Can you work these out from the model? Positions are in its coordinate system, mm. Face numbers are marked on the shaded views. A direction names the side the tool comes from. Round coordinates to 2 decimals unless told otherwise and drop trailing zeros. Loops run counter-clockwise (first coordinate to the right, second up) from the corner with the lowest first, then second, coordinate; pieces in that order, holes last. Notation, with made-up numbers: (75, -19.75) -> (96, -19.75) arc R20 ccw to (96, 13.25) -> close; hole circle Ø4 at (19.5, 16.25). An arc over 180 degrees is marked (long way). Write item = value, one per line.
from build123d import *

# Parameters (mm, degrees)
SKETCH2_R          = 3
EXTRUDE1_DEPTH     = 10
SKETCH3_R          = 5
EXTRUDE2_DEPTH     = 6
CUT_EXTRUDE1_DEPTH = 6
FILLET1_R          = 0.5
CHAMFER1_SIZE      = 0.5


with BuildPart() as part:
    # Sketch2 → Extrude1 (new body)
    with BuildSketch(Plane.XY):
        Circle(SKETCH2_R)
    extrude(amount=-EXTRUDE1_DEPTH)

    # Sketch3 → Extrude2 (add)
    with BuildSketch(Plane.XY):
        Circle(SKETCH3_R)
    extrude(amount=EXTRUDE2_DEPTH)

    # Sketch4 → Cut-Extrude1 (cut)
    with BuildSketch(Plane.XY.offset(6)):
        Polygon((-2.46568884, 1.501236783), (-2.532953611, -1.384730781), (-0.067264771, -2.885967565), (2.46568884, -1.501236783), (2.532953611, 1.384730781), (0.067264771, 2.885967565), align=None)
    extrude(amount=-CUT_EXTRUDE1_DEPTH, mode=Mode.SUBTRACT)

    # Fillet1
    fillet1_edges = [part.edges().sort_by_distance(p)[0] for p in [
        (-5, 0, 6),
    ]]
    fillet(fillet1_edges, radius=FILLET1_R)

    # Chamfer1
    chamfer1_edges = [part.edges().sort_by_distance(p)[0] for p in [
        (-1.199212034, 2.193602174, 6),
        (-2.499321225, 0.058253001, 6),
        (-1.300109191, -2.135349173, 6),
        (1.199212034, -2.193602174, 6),
        (2.499321225, -0.058253001, 6),
        (1.300109191, 2.135349173, 6),
    ]]
    chamfer(chamfer1_edges, length=CHAMFER1_SIZE)


solid = part.part
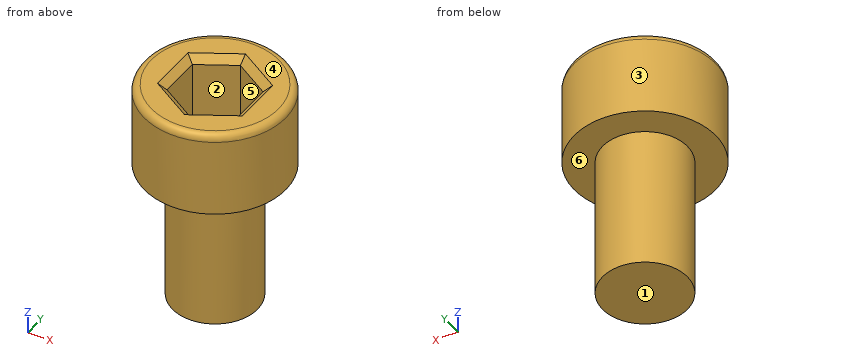
1. Suppose I cut it at A-A, the plane z = 3.75. List the corners of the cut face in (x, y) for me, and give its area (3 significant figures).
Entries:
outline = circle Ø10 at (0, 0); hole (-2.53, -1.38) -> (-0.07, -2.89) -> (2.47, -1.5) -> (2.53, 1.38) -> (0.07, 2.89) -> (-2.47, 1.5) -> close
area = 56.9 mm²
2. Suppose I cut it at C-C, the plane z = -4.25. List the corners of the cut face in (x, y) for me.
Entries:
outline = circle Ø6 at (0, 0)
3. I'm going to push flat-ended pins straight in: pin 1 (1.5 mm diameter, centred on y = -2.5, z = 4.5, fed in from -X); pin 2 (1 mm diameter, centred on x = -1.5, y = 4, fed in from -Z); pin 3 (1.5 mm diameter, centred on x = 0, y = 0.5, fed in from +Z). Where does each tip first touch, or does it pass through?
Entries:
pin_1 = -4.68
pin_2 = 0
pin_3 = 0
4. I need wall thicknesses on line 1 (Z direction, x = 0, y = -3.5); line 2 (Y direction, x = 4, z = 5); line 3 (X direction, y = -2.5, z = -1.5). Which ranges of each line are inside material? Lowest first, please. Write a range as [from, to].
Entries:
line_1 = [0, 6]
line_2 = [-3, 3]
line_3 = [-1.66, 1.66]
5. For the marked faces 4, 5 and 6, which set-ups out of +Z, -Z, +X, -X, +Y, -Y let a thin tool reach every point of the face, with its end or its side?
Entries:
face_4 = +Z, +X, -X, +Y, -Y
face_5 = +Z
face_6 = -Z
6. We'd pull the mould along X, two halves only. Please class the marked faces 1, 2 and 3: released by +X, released by -X, zero draft, split by the parting line, or undercut.
Entries:
face_1 = zero draft
face_2 = undercut
face_3 = split by the parting line
7. Suppose I cut it at B-B, the plane y = 0. List the corners of the cut face in (x, z) for me.
Entries:
outline = (-5, 0) -> (-3, 0) -> (-3, -10) -> (3, -10) -> (3, 0) -> (5, 0) -> (5, 5.5) arc R0.5 ccw to (4.5, 6) -> (3, 6) -> (2.5, 5.5) -> (2.5, 0) -> (-2.5, 0) -> (-2.5, 5.5) -> (-3, 6) -> (-4.5, 6) arc R0.5 ccw to (-5, 5.5) -> close
